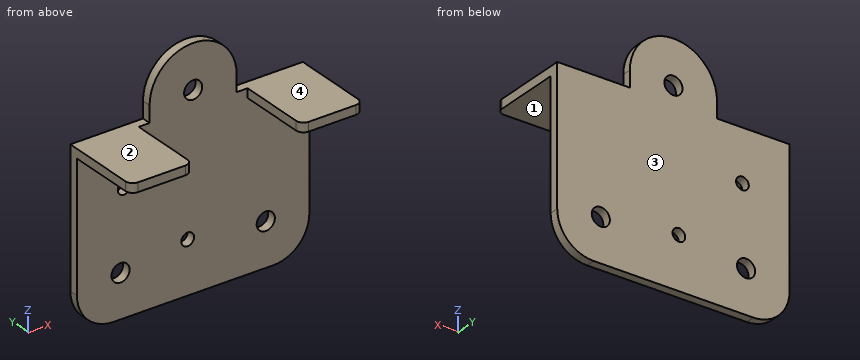
```python
from build123d import *

# Parameters (mm, degrees)
SKETCH2_W           = 64
SKETCH2_H           = 47.5
SKETCH2_R           = 1.75
BOSS_EXTRUDE1_DEPTH = 2.5
FILLET1_R           = 10
SKETCH3_R           = 2.5
BOSS_EXTRUDE2_DEPTH = 2.5
SKETCH4_W           = 17
SKETCH4_H           = 2.5
BOSS_EXTRUDE3_DEPTH = 20.4
FILLET2_R           = 2
SKETCH5_R           = 2.5
CUT_EXTRUDE1_DEPTH  = 23.9


with BuildPart() as part:
    # Sketch2 → Boss-Extrude1 (new body)
    with BuildSketch(Plane(origin=(0, 0, 0), x_dir=(1, 0, 0), z_dir=(0, 1, 0))):
        Rectangle(SKETCH2_W, SKETCH2_H)
        with Locations((-1.5, 9.4)):
            Circle(SKETCH2_R, mode=Mode.SUBTRACT)
        with Locations((-19, -9.5)):
            Circle(SKETCH2_R, mode=Mode.SUBTRACT)
    extrude(amount=BOSS_EXTRUDE1_DEPTH)

    # Fillet1
    fillet1_edges = [part.edges().sort_by_distance(p)[0] for p in [
        (-32, 1.25, -23.75),
        (32, 1.25, -23.75),
    ]]
    fillet(fillet1_edges, radius=FILLET1_R)

    # Sketch3 → Boss-Extrude2 (add)
    with BuildSketch(Plane(origin=(0, 2.5, 0), x_dir=(1, 0, 0), z_dir=(0, 1, 0))):
        with BuildLine():
            Line((-12, -28.25), (-12, -23.75))
            Line((-12, -23.75), (12, -23.75))
            Line((12, -23.75), (12, -28.25))
            ThreePointArc((12, -28.25), (0, -40.25), (-12, -28.25))
        make_face()
        with Locations((0, -28.25)):
            Circle(SKETCH3_R, mode=Mode.SUBTRACT)
    extrude(amount=-BOSS_EXTRUDE2_DEPTH)

    # Sketch4 → Boss-Extrude3 (add)
    with BuildSketch(Plane.XZ):
        with Locations((-23.5, 22.5)):
            Rectangle(SKETCH4_W, SKETCH4_H)
        with Locations((23.5, 22.5)):
            Rectangle(SKETCH4_W, SKETCH4_H)
    extrude(amount=BOSS_EXTRUDE3_DEPTH)

    # Fillet2
    fillet2_edges = [part.edges().sort_by_distance(p)[0] for p in [
        (-32, -20.4, 22.5),
        (-15, -20.4, 22.5),
        (32, -20.4, 22.5),
        (15, -20.4, 22.5),
    ]]
    fillet(fillet2_edges, radius=FILLET2_R)

    # Sketch5 → Cut-Extrude1 (cut, through all)
    with BuildSketch(Plane(origin=(0, 2.5, 0), x_dir=(1, 0, 0), z_dir=(0, 1, 0))):
        with Locations((-20, 11.85)):
            Circle(SKETCH5_R)
        with Locations((20, 11.85)):
            Circle(SKETCH5_R)
    extrude(amount=-CUT_EXTRUDE1_DEPTH, mode=Mode.SUBTRACT)


solid = part.part
```
Input: part model. Units: mm. Frame: model coordinates. Face numbers are marked on the shaded views. A direction names the side the tool comes from. Give positions to 0.01 mm unless a question says otherwise; leave off trailing zeros. Write each loop counter-clockwise with the first axis right and the second up, starting at its lowest first coordinate (ties: lowest second). Pieces come first, ordered by that corner, then holes. Notation, with made-up numbers: (-11, -8) - (24, -8) arc R8 ccw to (24, -4) - close; hole circle Ø7 at (-32.5, 30). An arc over 180 degrees is marked (long way). Write item = value, one per line. Start each with the question number.
1. Section query A-A, the plane x = 20. Output: boundary loops of the cut face in (y, z).
2. Section query C-C, the plane z = 9.5. Output: boundary loops of the cut face in (x, y).
3. Ray query, L1, parallel to X at y = 1.6, z = 28.25; L2, parallel to Z at x = -1.5, y = 1.1; L3, parallel to Y at x = -29, z = -12. Return the intervals inside material, ascending.
4. First-contact query: pin 1 Ø10 at (x, y) = (20.5, -15.5) entering from -Z; pin 2 Ø2 at (x, z) = (-24.5, 12.5) entering from -Y; pin 3 Ø0.8 at (y, z) = (0.5, 26) entering from +X. Flat tips, straight axial feed; report the tip coordinate or a pass-through.
5. Section query B-B, the plane y = -12.75. Output: boundary loops of the cut face in (x, z).
6. Section query D-D, the plane x = -19. Output: boundary loops of the cut face in (y, z).
7. Access query for the marked faces 1, 2, 3 and 4. Directions: +Z, -Z, +X, -X, +Y, -Y. A direction counts if a zero-diameter tool reaches every point of the face in a straight line with its end or side. Return the directions, or none.
Check sheet entries:
q1.outline = (-20.4, 21.25) - (0, 21.25) - (0, -9.35) - (2.5, -9.35) - (2.5, 23.75) - (-20.4, 23.75) - close; (0, -23.75) - (2.5, -23.75) - (2.5, -14.35) - (0, -14.35) - close
q2.outline = (-32, 0) - (-20.75, 0) - (-20.75, 2.5) - (-32, 2.5) - close; (-17.25, 0) - (32, 0) - (32, 2.5) - (-17.25, 2.5) - close
q3.L1 = -12 to -2.5, 2.5 to 12
q3.L2 = -23.75 to -11.15, -7.65 to 26.25, 30.25 to 40.16
q3.L3 = 0 to 2.5
q4.pin_1 = 21.25
q4.pin_2 = 0
q4.pin_3 = 12
q5.outline = (-32, 21.25) - (-15, 21.25) - (-15, 23.75) - (-32, 23.75) - close; (15, 21.25) - (32, 21.25) - (32, 23.75) - (15, 23.75) - close
q6.outline = (-20.4, 21.25) - (0, 21.25) - (0, 11.25) - (2.5, 11.25) - (2.5, 23.75) - (-20.4, 23.75) - close; (0, -23.75) - (2.5, -23.75) - (2.5, -14.14) - (0, -14.14) - close; (0, -9.56) - (2.5, -9.56) - (2.5, 7.75) - (0, 7.75) - close
q7.face_1 = -Z, +X, -X, -Y
q7.face_2 = +Z, -X, +Y, -Y
q7.face_3 = +Z, -Z, +X, -X, +Y
q7.face_4 = +Z, +X, +Y, -Y
